from build123d import *

# Parameters (mm, degrees)
F1_DEPTH = 581.025
F2_W     = 323.85
F2_H     = 114.3
F2_H_2   = 190.5
F2_W_2   = 336.55
F3_DEPTH = 565.15


with BuildPart() as f1:
    # F0 (on Front) → F1 (new body)
    with BuildSketch(Plane.XZ):
        Polygon((0, 361.95), (0, 0), (1422.4, 0), (1422.4, 361.95), (1060.45, 361.95), (1060.45, 228.6), (361.95, 228.6), (361.95, 361.95), align=None)
    extrude(amount=F1_DEPTH)

    # F2 (on face) → F3 (cut)
    with BuildSketch(Plane.XZ.offset(581.025)):
        with Locations((180.975, 285.75)):
            Rectangle(F2_W, F2_H)
        with Locations((180.975, 114.3)):
            Rectangle(F2_W, F2_H_2)
        with Locations((530.225, 114.3)):
            Rectangle(F2_W_2, F2_H_2)
        with Locations((892.175, 114.3)):
            Rectangle(F2_W_2, F2_H_2)
        with Locations((1241.425, 114.3)):
            Rectangle(F2_W, F2_H_2)
        with Locations((1241.425, 285.75)):
            Rectangle(F2_W, F2_H)
    extrude(amount=-F3_DEPTH, mode=Mode.SUBTRACT)


solid = f1.part
Source: CAD feature listing. Evaluate the final solid. Frame: model axes, mm. A direction names the side the tool comes from. Coordinates: 2 decimals unless noted, no trailing zeros. Loops run counter-clockwise (first coordinate to the right, second up) from the corner with the lowest first, then second, coordinate; pieces in that order, holes last. Notation, with made-up numbers: M -12,15 L 28,15 A25 cw 28,36 Z; hole C 22,-34.5 d5. An arc over 180 degrees is marked long. Answer in a Markdown table with one row per item.
Q1. First-contact query: pin 1 (4 mm diameter, centred on x = 693.5, y = -356.5, fed in from +Z); pin 2 (12 mm diameter, centred on x = 401, z = 105, fed in from -Y) (3 decimals). Flat tips, straight axial feed; report the tip coordinate or a pass-through.
Answers below:
| item | result |
|---|---|
| pin 1 | stops at z = 228.6 |
| pin 2 | stops at y = -15.875 |
Q2. Ray query, probe 1 along X at (y, z) = (-416.5, 191.5); probe 2 along Z at (x, y) = (129.5, -376.5); probe 3 along X at (y, z) = (-32, 297). Return the intervals inside material, ascending. Write a range as from..to.
Answers below:
| item | result |
|---|---|
| probe 1 | x = 0..19.05, 342.9..361.95, 698.5..723.9, 1060.45..1079.5, 1403.35..1422.4 |
| probe 2 | z = 0..19.05, 209.55..228.6, 342.9..361.95 |
| probe 3 | x = 0..19.05, 342.9..361.95, 1060.45..1079.5, 1403.35..1422.4 |
Q3. Set-up query: faces 1 (the flat face through (698.5, -302, 113)), 2 (the flat face through (1422.4, -286, 178)), 3 (the flat face through (716, -286, 228.6)). Return all of +Z, -Z, +X, -X, +Y, -Y with unobstructed straight access to the full face (end or side cutting, diameter ignored); none if empty.
Answers below:
| item | result |
|---|---|
| face 1 | -Y |
| face 2 | +Z, -Z, +X, +Y, -Y |
| face 3 | +Z, +Y, -Y |
Q4. Section D-D on z = 129.5. Return the cut outline in (x, y) (3 decimals), plus the area to 3 significant figures.
Answers below:
| item | result |
|---|---|
| outline | M 0,-581.025 L 19.05,-581.025 L 19.05,-15.875 L 342.9,-15.875 L 342.9,-581.025 L 361.95,-581.025 L 361.95,-15.875 L 698.5,-15.875 L 698.5,-581.025 L 723.9,-581.025 L 723.9,-15.875 L 1060.45,-15.875 L 1060.45,-581.025 L 1079.5,-581.025 L 1079.5,-15.875 L 1403.35,-15.875 L 1403.35,-581.025 L 1422.4,-581.025 L 1422.4,0 L 0,0 Z |
| area | 80,000 mm^2 |
Q5. Draft query along X for faces 4 (the flat face through (361.95, -286, 294)), 5 (the flat face through (0, -286, 184)), 6 (the flat face through (761, -581.025, 222)). Return one class per face: pulls with the +X half, pulls with the -X half, needs draft (parallel to the pull), parting line crosses it, or undercut.
Answers below:
| item | result |
|---|---|
| face 4 | undercut |
| face 5 | pulls with the -X half |
| face 6 | needs draft |
Q6. Section B-B on z = 268. Return the cut outline in (x, y) (3 decimals), plus the area to 3 significant figures.
Answers below:
| item | result |
|---|---|
| outline | M 0,-581.025 L 19.05,-581.025 L 19.05,-15.875 L 342.9,-15.875 L 342.9,-581.025 L 361.95,-581.025 L 361.95,0 L 0,0 Z; M 1060.45,-581.025 L 1079.5,-581.025 L 1079.5,-15.875 L 1403.35,-15.875 L 1403.35,-581.025 L 1422.4,-581.025 L 1422.4,0 L 1060.45,0 Z |
| area | 54,600 mm^2 |
Q7. Section A-A on x = 1262.5. Return the cut outline in (y, z) (3 decimals), plus the area to 3 significant figures.
Answers below:
| item | result |
|---|---|
| outline | M -581.025,0 L 0,0 L 0,361.95 L -581.025,361.95 L -581.025,342.9 L -15.875,342.9 L -15.875,228.6 L -581.025,228.6 L -581.025,209.55 L -15.875,209.55 L -15.875,19.05 L -581.025,19.05 Z |
| area | 38,000 mm^2 |
Q8. Section C-C on y = -542.5. State how many separate pieces and enclosed holes the cut face has, plus the area to 3 significant figures.
Answers below:
| item | result |
|---|---|
| separate pieces | 1 |
| enclosed holes | 6 |
| area | 96,000 mm^2 |
